Study the drawing (mm; zero at the part's minimum x, y, z) and answer. Coordinates: 2 decimals unless noted, no trailing zeros. Loops run counter-clockwise (first coordinate to the right, second up) from the corner with the lowest first, then second, coordinate; pieces in that order, holes last.
Q1. Straight lines are drawn through the part: line 1 (X direction, y = 3.25, z = 0.8); line 2 (X direction, y = 1, z = 1.35); line 3 (Y direction, x = 13, z = 0.25) (1 decimal). For each, find the intervals that lie inside material, in ascending order.
Q2. Flat-ended cylindrical pins translate along their axes: P1, Ø0.6, axis at x = 1.5, z = 1.5, coming from the -Y side; P2, Ø1, axis at y = 1, z = 1, coming from the -X side; P3, Ø1, axis at x = 5, z = 0.5, coming from the -Y side. Find the tip coordinate at first contact, or state that the pin passes through.
Q3. Section C-C (x = 52) is taken. Give the vertices of the cut face in (y, z).
Q4. Section D-D (y = 9) is taken. Give the vertices of the cut face in (x, z).
Q5. Section A-A (y = 4.25) is taken. Give the vertices of the cut face in (x, z).
Q6. Section B-B (z = 0.7) is taken. Give the vertices of the cut face in (x, y), then the cut area to 3 significant figures.
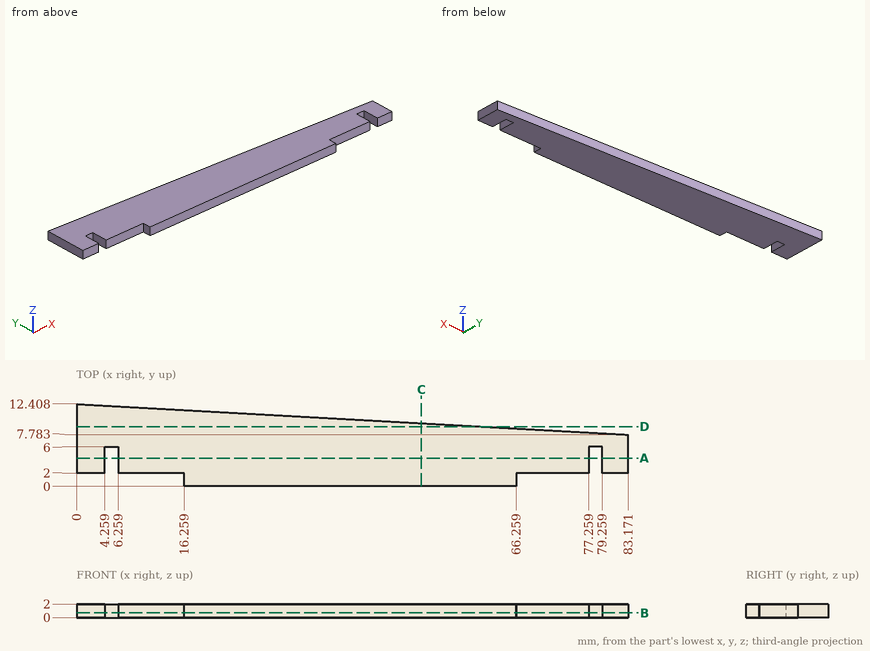
Numbers:
1. line 1: x = 0 to 4.26, 6.26 to 77.26, 79.26 to 83.17
1. line 2: x = 16.26 to 66.26
1. line 3: y = 2 to 11.7
2. P1: stops at y = 2
2. P2: stops at x = 16.26
2. P3: stops at y = 6
3. outline: (0, 0) - (9.52, 0) - (9.52, 2) - (0, 2) - close
4. outline: (0, 0) - (61.28, 0) - (61.28, 2) - (0, 2) - close
5. outline: (0, 0) - (4.26, 0) - (4.26, 2) - (0, 2) - close; (6.26, 0) - (77.26, 0) - (77.26, 2) - (6.26, 2) - close; (79.26, 0) - (83.17, 0) - (83.17, 2) - (79.26, 2) - close
6. outline: (0, 2) - (4.26, 2) - (4.26, 6) - (6.26, 6) - (6.26, 2) - (16.26, 2) - (16.26, 0) - (66.26, 0) - (66.26, 2) - (77.26, 2) - (77.26, 6) - (79.26, 6) - (79.26, 2) - (83.17, 2) - (83.17, 7.78) - (0, 12.41) - close
6. area: 757 mm2
